Can you work these out from the model? Positions are in its coordinate system, mm. Coordinates: 2 decimals unless noted, no trailing zeros. Order: outer loops, then holes, each group sorted by start corner. A loop starts at its lowest first (then second) coordinate and runs counter-clockwise, first axis right, second up. Notation, with made-up numbers: (1, -32) -> (5, -32) arc R5 ccw to (5, -24) -> close; hole circle Ø6 at (-38, -16.75). An arc over 180 degrees is marked (long way). Answer as CSV lines item,"result".
from build123d import *

# Parameters (mm, degrees)
F0_W     = 473.075
F0_H     = 341.3125
F0_R     = 2.15265
F0_R_2   = 1.7272
F0_W_2   = 41.275
F0_H_2   = 41.275
F1_DEPTH = 3.175
F3_R     = 4.7625
F2_R     = 1.7272
F4_DEPTH = 3.175
F5_R     = 1.7272
F6_DEPTH = 3.175


with BuildPart() as f1:
    # F0 (on Top) → F1 (new body)
    with BuildSketch(Plane.XY):
        Rectangle(F0_W, F0_H)
        with Locations((-128.679393, -62.798143)):
            Circle(F0_R, mode=Mode.SUBTRACT)
        with Locations((-119.167743, -63.302274)):
            Circle(F0_R_2, mode=Mode.SUBTRACT)
        with Locations((119.167743, -63.302274)):
            Circle(F0_R_2, mode=Mode.SUBTRACT)
        with Locations((128.679393, -62.798143)):
            Circle(F0_R, mode=Mode.SUBTRACT)
        with Locations((-196.85, 72.23125)):
            Circle(F0_R_2, mode=Mode.SUBTRACT)
        with Locations((-128.679393, 62.798143)):
            Circle(F0_R, mode=Mode.SUBTRACT)
        with Locations((-119.167743, 63.302274)):
            Circle(F0_R_2, mode=Mode.SUBTRACT)
        with Locations((-138.1125, 72.23125)):
            Circle(F0_R_2, mode=Mode.SUBTRACT)
        with Locations((-167.48125, 101.6)):
            Rectangle(F0_W_2, F0_H_2, mode=Mode.SUBTRACT)
        with Locations((-196.85, 130.96875)):
            Circle(F0_R_2, mode=Mode.SUBTRACT)
        with Locations((-138.1125, 130.96875)):
            Circle(F0_R_2, mode=Mode.SUBTRACT)
        with Locations((119.167743, 63.302274)):
            Circle(F0_R_2, mode=Mode.SUBTRACT)
        with Locations((128.679393, 62.798143)):
            Circle(F0_R, mode=Mode.SUBTRACT)
    extrude(amount=F1_DEPTH)

    # F3
    f3_edges = [f1.edges().sort_by_distance(p)[0] for p in [
        (236.5375, -170.65625, 1.5875),
        (236.5375, 170.65625, 1.5875),
        (-236.5375, 170.65625, 1.5875),
        (-236.5375, -170.65625, 1.5875),
    ]]
    fillet(f3_edges, radius=F3_R)

    # F2 (on face) → F4 (cut, through all)
    with BuildSketch(Plane.XY.offset(3.175)):
        with Locations((-206.375, -140.49375)):
            Circle(F2_R)
        with Locations((-206.375, 140.49375)):
            Circle(F2_R)
        with Locations((206.375, 140.49375)):
            Circle(F2_R)
        with Locations((206.375, -140.49375)):
            Circle(F2_R)
    extrude(amount=-F4_DEPTH, mode=Mode.SUBTRACT)

    # F5 (on face) → F6 (cut, through all)
    with BuildSketch(Plane.XY.offset(3.175)):
        with Locations((-134.937486, 0)):
            Circle(F5_R)
        with Locations((-204.7875, 0)):
            Circle(F5_R)
    extrude(amount=-F6_DEPTH, mode=Mode.SUBTRACT)


solid = f1.part
Q1. Imagine slicing it at B-B (x = -162). List the corners of the cut face in (y, z) for me (1 decimal), and give its area (3 significant figures).
Solution:
outline,"(-170.7, 0) -> (81, 0) -> (81, 3.2) -> (-170.7, 3.2) -> close; (122.2, 0) -> (170.7, 0) -> (170.7, 3.2) -> (122.2, 3.2) -> close"
area,"953 mm2"
Q2. If I drill on line 1 (Y direction, x = -196.85, z = 1.35); line 2 (Y direction, x = -160, z = 1.3); line 3 (X direction, y = 116, z = 1.05), over which ranges is the centre line in solid material (lowest first)?
Solution:
line 1,"-170.66 to 70.5, 73.96 to 129.24, 132.7 to 170.66"
line 2,"-170.66 to 80.96, 122.24 to 170.66"
line 3,"-236.54 to -188.12, -146.84 to 236.54"
Q3. Imagine slicing it at A-A (y = 98). List the corners of the cut face in (x, z) for me (1 decimal), and give its area (3 significant figures).
Solution:
outline,"(-236.5, 0) -> (-188.1, 0) -> (-188.1, 3.2) -> (-236.5, 3.2) -> close; (-146.8, 0) -> (236.5, 0) -> (236.5, 3.2) -> (-146.8, 3.2) -> close"
area,"1,370 mm2"
